from build123d import *

# Parameters (mm, degrees)
BOSS_EXTRUDE1_DEPTH = 231.775
SKETCH2_R           = 3.2639
CUT_EXTRUDE1_DEPTH  = 12.7
SKETCH3_R           = 3.2639
CUT_EXTRUDE2_DEPTH  = 12.7


with BuildPart() as part:
    # Sketch1 → Boss-Extrude1 (new body)
    with BuildSketch(Plane(origin=(0, 0, 0), x_dir=(0, 0, -1), z_dir=(1, 0, 0))):
        Polygon((0, 7.332348419), (-6.35, 3.666174209), (-6.35, -3.666174209), (0, -7.332348419), (6.35, -3.666174209), (6.35, 3.666174209), align=None)
    extrude(amount=BOSS_EXTRUDE1_DEPTH)

    # Sketch2 → Cut-Extrude1 (cut)
    with BuildSketch(Plane(origin=(231.775, 0, 0), x_dir=(0, 0, -1), z_dir=(1, 0, 0))):
        Circle(SKETCH2_R)
    extrude(amount=-CUT_EXTRUDE1_DEPTH, mode=Mode.SUBTRACT)

    # Sketch3 → Cut-Extrude2 (cut)
    with BuildSketch(Plane.ZY):
        Circle(SKETCH3_R)
    extrude(amount=-CUT_EXTRUDE2_DEPTH, mode=Mode.SUBTRACT)


solid = part.part
Verification items for the finished model (mm, model axes). A direction names the side the tool comes from. Round coordinates to 2 decimals unless told otherwise and drop trailing zeros. Write each loop counter-clockwise with the first axis right and the second up, starting at its lowest first coordinate (ties: lowest second). Pieces come first, ordered by that corner, then holes.
(1) Section check B-B (x = 107.5). Enter the section's corners in (y, z), plus the area to 3 significant figures.
Returned:
outline: (-7.33, 0) - (-3.67, -6.35) - (3.67, -6.35) - (7.33, 0) - (3.67, 6.35) - (-3.67, 6.35) - close
area: 140 mm2
(2) Depth check by flat-ended pin: pin 1 Ø4 at (y, z) = (0, 0) entering from +X (3 decimals); pin 2 Ø1 at (x, z) = (27.5, -3) entering from -Y; pin 3 Ø3 at (x, z) = (136, 4.5) entering from -Y. Enter the tip coordinate at first touch or a pass-through.
Returned:
pin 1: stops at x = 219.075
pin 2: stops at y = -5.89
pin 3: stops at y = -5.6
(3) Material ranges on line 1 (Y direction, x = 225, z = 0); line 2 (X direction, y = -1, z = -3) (3 decimals); line 3 (Y direction, x = 54.5, z = -1.75), recorded low to high.
Returned:
line 1: y = -7.33 to -3.26, 3.26 to 7.33
line 2: x = 12.7 to 219.075
line 3: y = -6.32 to 6.32
(4) Mould release check, pull along Y, two halves, no side actions. Record for faces 1 (the flat face through (114.265, 5.474, -3.219)), 2 (the cylindrical face through (6.261, -3.186, -0.708)), 3 (the flat face through (0, -2, 3)): pulls with the +Y half, pulls with the -Y half, needs draft (parallel to the pull), parting line crosses it, or undercut.
Returned:
face 1: pulls with the +Y half
face 2: undercut
face 3: needs draft
(5) Access from +Z, -Z, +X, -X, +Y, -Y to the whole of each face (thin tool, end or side, straight path). Record for faces 4 (the flat face through (12.7, 0, 0)), 5 (the flat face through (114, 0, -6.35)), 6 (the flat face through (219.075, 0, 0)).
Returned:
face 4: -X
face 5: -Z, +X, -X, +Y, -Y
face 6: +X
(6) Section check A-A (y = 0). Enter the section's corners in (x, z) (3 decimals).
Returned:
outline: (0, -6.35) - (231.775, -6.35) - (231.775, -3.264) - (219.075, -3.264) - (219.075, 3.264) - (231.775, 3.264) - (231.775, 6.35) - (0, 6.35) - (0, 3.264) - (12.7, 3.264) - (12.7, -3.264) - (0, -3.264) - close
